Can you work these out from the model? Positions are in its coordinate system, mm. Face numbers are marked on the shaded views. A direction names the side the tool comes from. Give positions to 0.01 mm unless a question says otherwise; leave off trailing zeros. Loops run counter-clockwise (first coordinate to the right, second up) from the corner with the lowest first, then second, coordinate; pieces in that order, holes last. Notation, with made-up numbers: (63, 10) - (84, 10) arc R20 cw to (84, 48) - close; hole circle Ø4 at (38, 84). An arc over 180 degrees is marked (long way). Answer as a JSON object with one key per item and string values. Group by question number.
Item 1: Suppose I cut it at B-B on z = -2.9. Write out the boundary of the cut face in (x, y).
Item 2: Please list where these lines run through material, in increasing order: L1, parallel to Y at x = 6.5, z = -0.6; L2, parallel to Y at x = 1.75, z = -1.7; L3, parallel to X at y = 16, z = -2.4.
Item 3: Suppose I cut it at C-C on x = 7.5. Write out the boundary of the cut face in (y, z), and give its area (3 significant figures).
Item 4: Will these pins go through, and if not, where does the flat tip stop? pin 1 (0.9 mm diameter, centred on x = 7, z = -2.5, fed in from -Y); pin 2 (2.5 mm diameter, centred on x = 8, z = -3.5, fed in from +Y); pin 3 (1.5 mm diameter, centred on y = 39, z = -3, fed in from +X).
Item 5: Thinking about a two-plate mould opening in Y: for the marked faces 1, 2, 3 and 4, which applies, pulls with the +Y half, pulls with the -Y half, needs draft (parallel to the pull), parting line crosses it, or undercut?
Item 6: Suppose I cut it at A-A on x = 1.5. Write out the boundary of the cut face in (y, z), and give its area (4 significant figures).
Item 7: Which directions (+Z, -Z, +X, -X, +Y, -Y) give clear straight access to the entire face, cutting with the end or side of a thin tool? Please do the marked faces 5, 6, 7, 8 and 9.
Item 8: Suppose I cut it at D-D on y = 27. Write out the boundary of the cut face in (x, z), and give its area (3 significant figures).
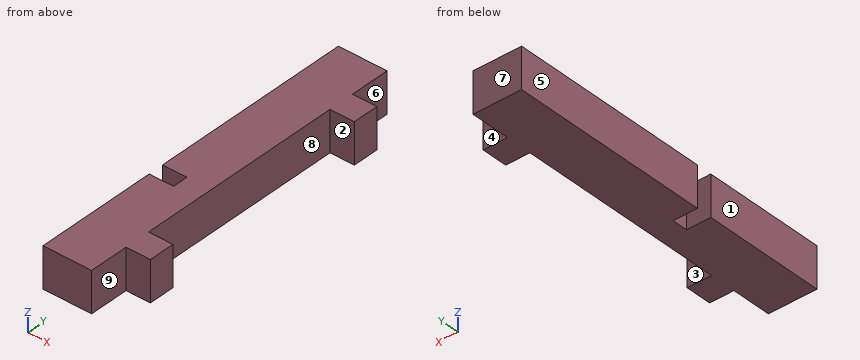
Autodesk Inventor part; units mm, degrees
ref_plane "YZ Plane" through (0, 0, 0) normal (1, 0, 0) x (0, 1, 0)
ref_plane "XZ Plane" through (0, 0, 0) normal (0, 1, 0) x (-1, 0, 0)
ref_plane "XY Plane" through (0, 0, 0) normal (0, 0, 1) x (1, 0, 0)
sketch "Sketch1" plane through (0, 0, 0) normal (0, 0, 1) x (1, 0, 0)
  line L0 (0, 42) -> (6, 42)
  line L1 (6, 42) -> (6, 0)
  line L2 (6, 0) -> (0, 0)
  line L3 (0, 0) -> (0, 42)
  dimension "d0" = 6
  dimension "d1" = 42
extrude "Extrusion1" add sketch "Sketch1" against normal blind 5
sketch "Sketch4" plane through (0, 0, 0) normal (0, 0, 1) x (1, 0, 0)
  line L0 (0, 0) -> (0, 42)
  line L1 (0, 17) -> (3, 17)
  line L2 (3, 17) -> (3, 15.1)
  line L3 (3, 15.1) -> (0, 15.1)
  line L4 (0, 15.1) -> (0, 17)
  line L5 (6, 0) -> (0, 0)
  point P0 (0, 45)
  dimension "d12" = 1.9
  dimension "d13" = 3
  dimension "d18" = 17
extrude "Extrusion4" cut sketch "Sketch4" against normal blind 5
sketch "Sketch5" plane through (0, 0, 0) normal (0, 0, 1) x (1, 0, 0)
  line L0 (6, 42) -> (6, 0)
  line L1 (6, 0) -> (0, 0)
  line L2 (0, 42) -> (6, 42)
  line L3 (6, 42) -> (6, 0)
  line L4 (9, 8.1) -> (6, 8.1)
  line L5 (6, 8.1) -> (6, 4.9)
  line L6 (6, 4.9) -> (9, 4.9)
  line L7 (9, 4.9) -> (9, 8.1)
  line L8 (9, 8.1) -> (6, 4.9) construction
  line L9 (6, 8.1) -> (9, 4.9) construction
  line L10 (9, 37.1) -> (6, 37.1)
  line L11 (6, 37.1) -> (6, 33.9)
  line L12 (6, 33.9) -> (9, 33.9)
  line L13 (9, 33.9) -> (9, 37.1)
  line L14 (9, 37.1) -> (6, 33.9) construction
  line L15 (6, 37.1) -> (9, 33.9) construction
  line L16 (0, 42) -> (6, 0) construction
  line L17 (0, 0) -> (6, 42) construction
  point P0 (7.5, 6.5)
  point P1 (7.5, 35.5)
  point P2 (3, 21)
  dimension "d31" = 3
  dimension "d32" = 3.2
  dimension "d34" = 14.5
  dimension "d35" = 14.5
  dimension "d36" = 3.2
extrude "Extrusion5" add sketch "Sketch5" against normal blind 5
equation "\"d36\" = d32"
equation "\"kerf\" = 0.15"
properties part number "PCBSupport"
Worked out:
{
 "1": {"outline": "(0, 0) - (6, 0) - (6, 4.9) - (9, 4.9) - (9, 8.1) - (6, 8.1) - (6, 33.9) - (9, 33.9) - (9, 37.1) - (6, 37.1) - (6, 42) - (0, 42) - (0, 17) - (3, 17) - (3, 15.1) - (0, 15.1) - close"},
 "2": {"L1": "y = 4.9 to 8.1, 33.9 to 37.1", "L2": "y = 0 to 15.1, 17 to 42", "L3": "x = 3 to 6"},
 "3": {"outline": "(4.9, -5) - (8.1, -5) - (8.1, 0) - (4.9, 0) - close; (33.9, -5) - (37.1, -5) - (37.1, 0) - (33.9, 0) - close", "area": "32.0 mm2"},
 "4": {"pin 1": "stops at y = 4.9", "pin 2": "stops at y = 37.1", "pin 3": "stops at x = 6"},
 "5": {"face 1": "needs draft", "face 2": "undercut", "face 3": "undercut", "face 4": "pulls with the +Y half"},
 "6": {"outline": "(0, -5) - (15.1, -5) - (15.1, 0) - (0, 0) - close; (17, -5) - (42, -5) - (42, 0) - (17, 0) - close", "area": "200.5 mm2"},
 "7": {"face 5": "+Z, -Z, -X, +Y, -Y", "face 6": "+Z, -Z, +X, +Y", "face 7": "+Z, -Z, +X, -X, +Y", "face 8": "+Z, -Z, +X", "face 9": "+Z, -Z, +X, -Y"},
 "8": {"outline": "(0, -5) - (6, -5) - (6, 0) - (0, 0) - close", "area": "30.0 mm2"}
}
